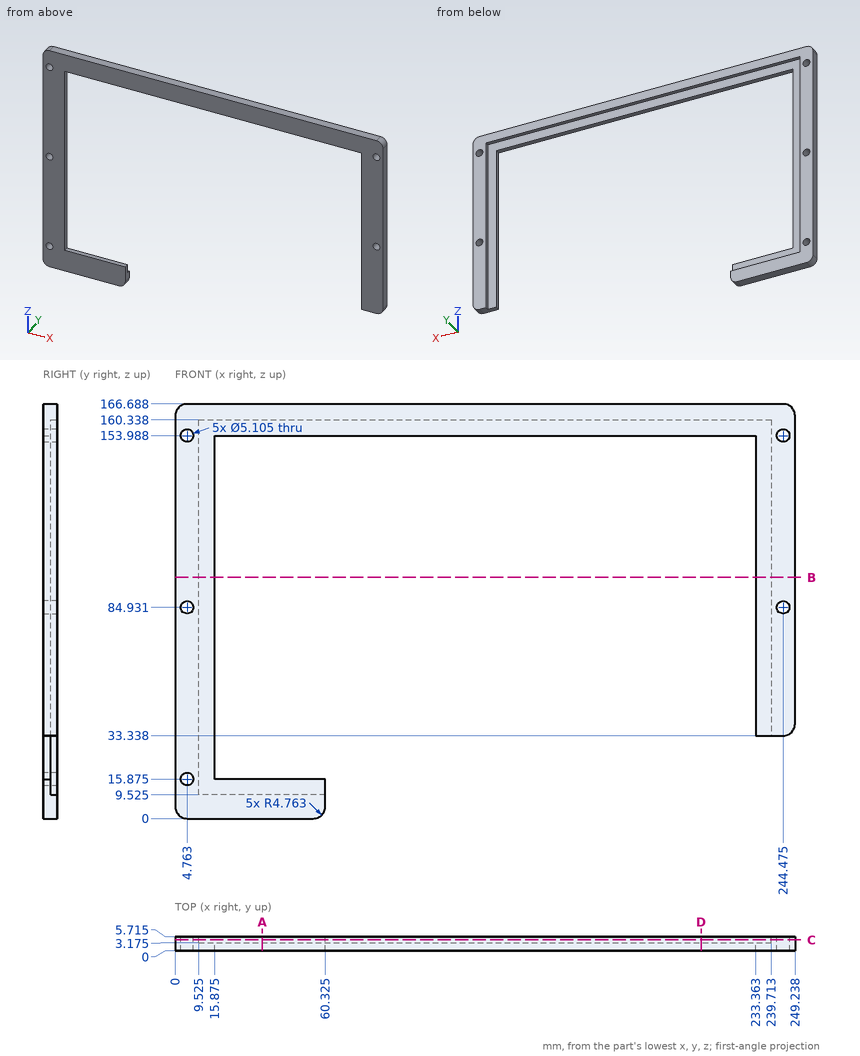
Input: dimensioned drawing with shaded views. Units: mm. Origin: part minimum x, y, z. Give positions to 0.01 mm unless a question says otherwise; leave off trailing zeros. Write each loop counter-clockwise with the first axis right and the second up, starting at its lowest first coordinate (ties: lowest second). Pieces come first, ordered by that corner, then holes.
1. First-contact query: pin 1 (3 mm diameter, centred on x = 241.5, y = 3, fed in from -Z); pin 2 (1.5 mm diameter, centred on x = 104.5, y = 3.5, fed in from -Z); pin 3 (4 mm diameter, centred on x = 244.48, z = 84.93, fed in from +Y); pin 4 (1.3 mm diameter, centred on x = 88, y = 5, fed in from -Z). Flat tips, straight axial feed; report the tip coordinate or a pass-through.
2. Section query C-C (y = 4.4). Return the cut outline in (x, z) (1 decimal).
3. Section query A-A (x = 35). Return the cut outline in (y, z) (1 decimal).
4. Material intervals for line 1 along X through (y, z) = (4.7, 54) (1 decimal); line 2 along X through (y, z) = (0.65, 50.5) (1 decimal); line 3 along Z through (x, y) = (46, 0.8) (1 decimal), sorted ascending.
5. Section query B-B (z = 97). Return the cut outline in (x, y) (1 decimal).
6. Section query D-D (x = 211.5). Return the cut outline in (y, z) (1 decimal).
Output values:
1. pin 1: stops at z = 33.34
1. pin 2: stops at z = 153.99
1. pin 3: passes through
1. pin 4: stops at z = 160.34
2. outline: (0, 4.8) arc R4.8 ccw to (4.8, 0) - (55.6, 0) arc R4.8 ccw to (60.3, 4.8) - (60.3, 9.5) - (9.5, 9.5) - (9.5, 160.3) - (239.7, 160.3) - (239.7, 33.3) - (244.5, 33.3) arc R4.8 ccw to (249.2, 38.1) - (249.2, 161.9) arc R4.8 ccw to (244.5, 166.7) - (4.8, 166.7) arc R4.8 ccw to (0, 161.9) - close; hole circle Ø5.1 at (4.8, 15.9); hole circle Ø5.1 at (4.8, 84.9); hole circle Ø5.1 at (4.8, 154); hole circle Ø5.1 at (244.5, 84.9); hole circle Ø5.1 at (244.5, 154)
3. outline: (0, 0) - (5.7, 0) - (5.7, 9.5) - (3.2, 9.5) - (3.2, 15.9) - (0, 15.9) - close; (0, 154) - (3.2, 154) - (3.2, 160.3) - (5.7, 160.3) - (5.7, 166.7) - (0, 166.7) - close
4. line 1: x = 0 to 9.5, 239.7 to 249.2
4. line 2: x = 0 to 15.9, 233.4 to 249.2
4. line 3: z = 0 to 15.9, 154 to 166.7
5. outline: (0, 0) - (15.9, 0) - (15.9, 3.2) - (9.5, 3.2) - (9.5, 5.7) - (0, 5.7) - close; (233.4, 0) - (249.2, 0) - (249.2, 5.7) - (239.7, 5.7) - (239.7, 3.2) - (233.4, 3.2) - close
6. outline: (0, 154) - (3.2, 154) - (3.2, 160.3) - (5.7, 160.3) - (5.7, 166.7) - (0, 166.7) - close
